Check sheet for the drawn part. Datum: minimum x, y, z corner. Units: mm. A direction names the side the tool comes from. Round coordinates to 2 decimals unless told otherwise and drop trailing zeros. Write each loop counter-clockwise with the first axis right and the second up, starting at its lowest first coordinate (ties: lowest second). Pieces come first, ordered by that corner, then holes.
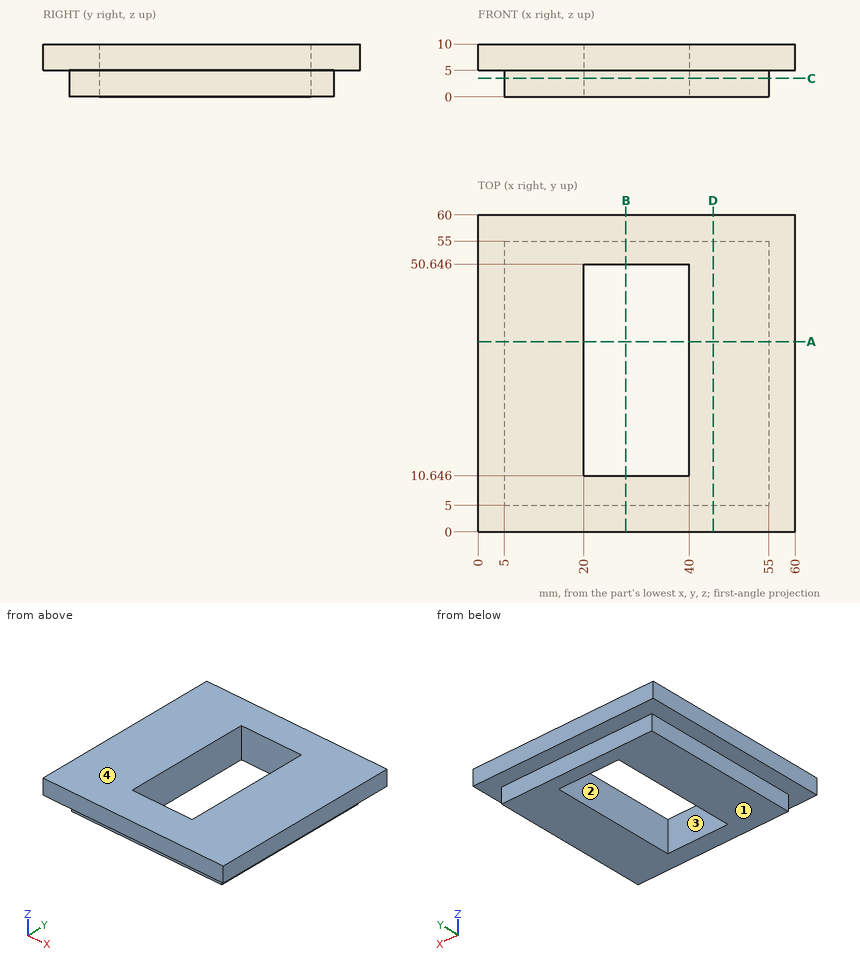
Q1. Sectioned sample at B-B (x = 28). Enter the section's corners in (y, z), plus the area to 3 significant figures.
Recorded:
outline: (0, 5) - (5, 5) - (5, 0) - (10.65, 0) - (10.65, 10) - (0, 10) - close; (50.65, 0) - (55, 0) - (55, 5) - (60, 5) - (60, 10) - (50.65, 10) - close
area: 150 mm2
Q2. Sectioned sample at C-C (z = 3.5). Enter the section's corners in (x, y).
Recorded:
outline: (5, 5) - (55, 5) - (55, 55) - (5, 55) - close; hole (20, 10.65) - (40, 10.65) - (40, 50.65) - (20, 50.65) - close
Q3. Release check for a two-part mould opening along X. For the marked faces 3 and 4 record: released by +X, released by -X, zero draft, split by the parting line, or undercut.
Recorded:
face 3: undercut
face 4: zero draft
Q4. Sectioned sample at A-A (y = 36). Enter the section's corners in (x, z), plus the area to 3 significant figures.
Recorded:
outline: (0, 5) - (5, 5) - (5, 0) - (20, 0) - (20, 10) - (0, 10) - close; (40, 0) - (55, 0) - (55, 5) - (60, 5) - (60, 10) - (40, 10) - close
area: 350 mm2
Q5. Depth check by flat-ended pin: P1, Ø1.5, axis at y = 32, z = 2.5, coming from the -X side; P2, Ø1.5, axis at y = 38, z = 3.5, coming from the +X side; P3, Ø2.5, axis at x = 24.5, z = 3.5, coming from the -Y side. Enter the tip coordinate at first touch or a pass-through.
Recorded:
P1: stops at x = 5
P2: stops at x = 55
P3: stops at y = 5
Q6. Tool access check on the marked faces 1 and 2. Record the directions out of +Z, -Z, +X, -X, +Y, -Y that give a thin tool (end or side, any length) a straight path to the whole face; none if there is none.
Recorded:
face 1: -Z, +X, -X, +Y, -Y
face 2: +Z, -Z
Q7. Sectioned sample at D-D (x = 44.5). Enter the section's corners in (y, z).
Recorded:
outline: (0, 5) - (5, 5) - (5, 0) - (55, 0) - (55, 5) - (60, 5) - (60, 10) - (0, 10) - close
Q8. Material ranges on line 1 along Y through (x, z) = (28, 1.75); line 2 along X through (y, z) = (30, 2); line 3 along X through (y, z) = (37, 6), recorded low to high.
Recorded:
line 1: y = 5 to 10.65, 50.65 to 55
line 2: x = 5 to 20, 40 to 55
line 3: x = 0 to 20, 40 to 60
